```python
from build123d import *

# Parameters (mm, degrees)
SKETCH1_R           = 25
BOSS_EXTRUDE3_DEPTH = 200
SKETCH3_R           = 21.5
CUT_EXTRUDE1_DEPTH  = 190
CUT_EXTRUDE2_REACH  = 202
SKETCH5_R           = 10
CUT_EXTRUDE3_REACH  = 27
SKETCH6_R           = 21.5


with BuildPart() as part:
    # Sketch1 → Boss-Extrude3 (new body)
    with BuildSketch(Plane(origin=(0, 0, 0), x_dir=(0, 0, -1), z_dir=(1, 0, 0))):
        Circle(SKETCH1_R)
    extrude(amount=BOSS_EXTRUDE3_DEPTH)

    # Sketch3 → Cut-Extrude1 (cut)
    with BuildSketch(Plane(origin=(200, 0, 0), x_dir=(0, 0, -1), z_dir=(1, 0, 0))):
        Circle(SKETCH3_R)
    extrude(amount=-CUT_EXTRUDE1_DEPTH, mode=Mode.SUBTRACT)

    # Sketch5 → Cut-Extrude2 (cut, up to next)
    with BuildSketch(Plane.ZY, mode=Mode.PRIVATE) as cut_extrude2_sk1:
        Circle(SKETCH5_R)
    cut_extrude2_tool1 = extrude(cut_extrude2_sk1.sketch, amount=-CUT_EXTRUDE2_REACH, mode=Mode.PRIVATE) & part.part
    add(cut_extrude2_tool1.solids().sort_by_distance((0, 0, 0))[0], mode=Mode.SUBTRACT)

    # Sketch6 → Cut-Extrude3 (cut, up to next)
    with BuildSketch(Plane(origin=(0, 0, 0), x_dir=(1, 0, 0), z_dir=(0, 1, 0)), mode=Mode.PRIVATE) as cut_extrude3_sk1:
        with Locations((86, 0)):
            Circle(SKETCH6_R)
    cut_extrude3_tool1 = extrude(cut_extrude3_sk1.sketch, amount=-CUT_EXTRUDE3_REACH, mode=Mode.PRIVATE) & part.part
    add(cut_extrude3_tool1.solids().sort_by_distance((86, 0, 0))[0], mode=Mode.SUBTRACT)


solid = part.part
```
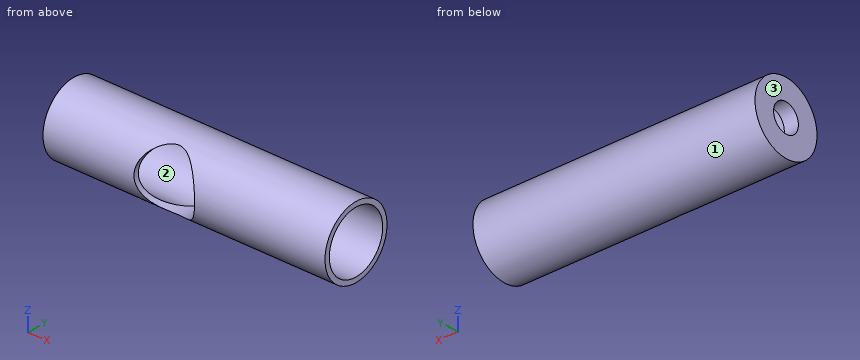
Here's how the part is built. I have some questions about the finished solid (model axes, mm). Face numbers are marked on the shaded views. Round coordinates to 2 decimals unless told otherwise and drop trailing zeros. Order: outer loops, then holes, each group sorted by start corner. A loop starts at its lowest first (then second) coordinate and runs counter-clockwise, first axis right, second up. Notation, with made-up numbers: M 80.25,89 L 91.25,89 A25 ccw 91.25,108 Z; hole C 29.5,78.5 d11. An arc over 180 degrees is marked long. Answer in a Markdown table with one row per item.
Item 1: Thinking about a two-plate mould opening in Y: for the marked faces 1, 2 and 3, which applies, +Y half, -Y half, draft (parallel to the pull), parting line (faces both ways), or undercut?
A:
| item | result |
|---|---|
| face 1 | parting line |
| face 2 | undercut |
| face 3 | draft |
Item 2: Imagine slicing it at D-D, the plane z = -17.5. Write out the boundary of the cut face in (x, y), and give its area (3 significant figures).
A:
| item | result |
|---|---|
| outline | M 0,-17.85 L 73.51,-17.85 L 73.51,-12.49 L 10,-12.49 L 10,12.49 L 200,12.49 L 200,17.85 L 0,17.85 Z; M 98.49,-17.85 L 200,-17.85 L 200,-12.49 L 98.49,-12.49 Z |
| area | 2,260 mm2 |
Item 3: Imagine slicing it at B-B, the plane y = -5. Write out the boundary of the cut face in (x, z).
A:
| item | result |
|---|---|
| outline | M 0,-24.49 L 200,-24.49 L 200,-20.91 L 91,-20.91 A21.5 cw 81,-20.91 L 10,-20.91 L 10,-8.66 L 0,-8.66 Z; M 0,8.66 L 10,8.66 L 10,20.91 L 81,20.91 A21.5 cw 91,20.91 L 200,20.91 L 200,24.49 L 0,24.49 Z |
Item 4: I'm going to push flat-ended pins straight in: pin 1 (5 mm diameter, centred on x = 58, y = 18, fed in from -Z); pin 2 (21.5 mm diameter, centred on y = 2, z = 9, fed in from +X); pin 3 (6 mm diameter, centred on x = 142, y = -16.5, fed in from -Z). Where does each tip first touch, or does it pass through?
A:
| item | result |
|---|---|
| pin 1 | stops at z = -19.62 |
| pin 2 | stops at x = 10 |
| pin 3 | stops at z = -21.04 |
Item 5: If I drill on L1, parallel to Y at x = 4, z = 0; L2, parallel to Z at x = 187.5, y = 1; L3, parallel to X at y = 4, z = -11.5, over which ranges is the centre line in solid material (lowest first)? Write a range as from..to.
A:
| item | result |
|---|---|
| L1 | y = -25..-10, 10..25 |
| L2 | z = -24.98..-21.48, 21.48..24.98 |
| L3 | x = 0..10 |
Item 6: Imagine slicing it at A-A, the plane z = 0. Write out the boundary of the cut face in (x, y), and give its area (3 significant figures).
A:
| item | result |
|---|---|
| outline | M 0,-25 L 64.5,-25 L 64.5,-21.5 L 10,-21.5 L 10,-10 L 0,-10 Z; M 0,10 L 10,10 L 10,21.5 L 200,21.5 L 200,25 L 0,25 Z; M 107.5,-25 L 200,-25 L 200,-21.5 L 107.5,-21.5 Z |
| area | 1,480 mm2 |
Item 7: Imagine slicing it at C-C, the plane x = 50. Write out the boundary of the cut face in (y, z).
A:
| item | result |
|---|---|
| outline | C 0,0 d50; hole C 0,0 d43 |
